```python
from build123d import *

# Parameters (mm, degrees)
EXTRUDE_THIN1_DEPTH = 285.75
FILLET1_R           = 0.889


with BuildPart() as part:
    # Sketch1 → Extrude-Thin1 (new body)
    with BuildSketch(Plane.XY):
        with BuildLine():
            Line((-0.396875, -9.525), (0, -14.2875))
            ThreePointArc((0, -14.2875), (-2.898897336, -13.767099717), (-5.435779046, -12.270886692))
            ThreePointArc((-5.435779046, -12.270886692), (-8.464256404, -10.6095065), (-11.90625, -10.31875))
            Line((-11.90625, -10.31875), (-11.90625, -8.73125))
            Line((-11.90625, -8.73125), (-14.2875, -8.73125))
            Line((-14.2875, -8.73125), (-14.2875, -4.7625))
            Line((-14.2875, -4.7625), (-1.285875, -5.55625))
            Line((-1.285875, -5.55625), (-1.285875, 5.55625))
            Line((-1.285875, 5.55625), (-14.2875, 4.7625))
            Line((-14.2875, 4.7625), (-14.2875, 8.73125))
            Line((-14.2875, 8.73125), (-11.90625, 8.73125))
            Line((-11.90625, 8.73125), (-11.90625, 10.31875))
            ThreePointArc((-11.90625, 10.31875), (-8.464256404, 10.6095065), (-5.435779046, 12.270886692))
            ThreePointArc((-5.435779046, 12.270886692), (-2.898897336, 13.767099717), (0, 14.2875))
            Line((0, 14.2875), (-0.396875, 9.525))
            Line((-0.396875, 9.525), (-1.282804179, 9.598827432))
            Line((-1.282804179, 9.598827432), (-0.971469005, 13.334849518))
            ThreePointArc((-0.971469005, 13.334849518), (-3.040522473, 12.749361604), (-4.855962615, 11.596992112))
            ThreePointArc((-4.855962615, 11.596992112), (-7.731844672, 9.916114382), (-11.01725, 9.366424127))
            Line((-11.01725, 9.366424127), (-11.01725, 7.84225))
            Line((-11.01725, 7.84225), (-13.3985, 7.84225))
            Line((-13.3985, 7.84225), (-13.3985, 5.707428664))
            Line((-13.3985, 5.707428664), (-0.396875, 6.501178664))
            Line((-0.396875, 6.501178664), (-0.396875, -6.501178664))
            Line((-0.396875, -6.501178664), (-13.3985, -5.707428664))
            Line((-13.3985, -5.707428664), (-13.3985, -7.84225))
            Line((-13.3985, -7.84225), (-11.01725, -7.84225))
            Line((-11.01725, -7.84225), (-11.01725, -9.366424127))
            ThreePointArc((-11.01725, -9.366424127), (-7.731844672, -9.916114382), (-4.855962615, -11.596992112))
            ThreePointArc((-4.855962615, -11.596992112), (-3.040522473, -12.749361604), (-0.971469005, -13.334849518))
            Line((-0.971469005, -13.334849518), (-1.282804179, -9.598827432))
            Line((-1.282804179, -9.598827432), (-0.396875, -9.525))
        make_face()
    extrude(amount=-EXTRUDE_THIN1_DEPTH)

    # Fillet1
    fillet1_edges = [part.edges().sort_by_distance(p)[0] for p in [
        (-11.90625, -10.31875, -142.875),
        (-14.2875, -8.73125, -142.875),
        (-14.2875, -4.7625, -142.875),
        (-14.2875, 4.7625, -142.875),
        (-14.2875, 8.73125, -142.875),
        (-11.90625, 10.31875, -142.875),
        (-11.01725, 7.84225, -142.875),
        (-0.396875, 6.501178664, -142.875),
        (-0.396875, -6.501178664, -142.875),
        (-11.01725, -7.84225, -142.875),
    ]]
    fillet(fillet1_edges, radius=FILLET1_R)


solid = part.part
```
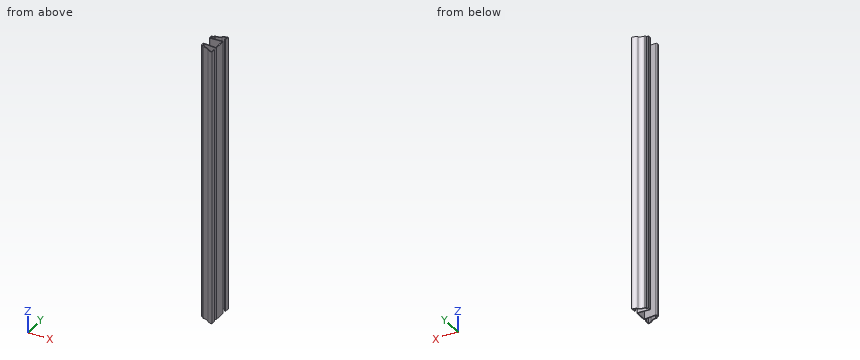
The listing builds one solid part. Answer for the finished solid, in the listing's coordinates (mm). Coordinates: 2 decimals unless noted, no trailing zeros. Order: outer loops, then holes, each group sorted by start corner. A loop starts at its lowest first (then second) coordinate and runs counter-clockwise, first axis right, second up. Notation, with made-up numbers: M -39.5,-35.5 L -26.5,-35.5 A14 ccw -26.5,-13.5 Z; hole C -32,-27.5 d2. An arc over 180 degrees is marked long. Answer as a JSON object with one key per item and string values. Group by question number.
1. Straight lines are drawn through the part: line 1 (Y direction, x = -3, z = -49.5); line 2 (Y direction, x = -2.25, z = -127.5); line 3 (X direction, y = 9, z = -29.5). For each, find the intervals that lie inside material, in ascending order.
2. Flat-ended cylindrical pins translate along their axes: P1, Ø8, axis at y = 3, z = -56.5, coming from the +X side; P2, Ø1.1, axis at y = 6.5, z = -122, coming from the +X side; P3, Ø1.2, axis at x = -13, z = -93, coming from the +Y side. Find the tip coordinate at first contact, or state that the pin passes through.
3. Section B-B on y = -0.5 is taken. Write down the section's boundary in (x, z).
4. Section A-A on x = -8.5 is taken. Write down the section's boundary in (y, z).
Values follow:
{
 "1": {"line 1": "-13.73 to -12.77, -6.34 to -5.45, 5.45 to 6.34, 12.77 to 13.73", "line 2": "-13.98 to -13.05, -6.39 to -5.5, 5.5 to 6.39, 13.05 to 13.98", "line 3": "-11.91 to -11.02"},
 "2": {"P1": "x = -0.4", "P2": "x = -0.49", "P3": "y = 8.73"},
 "3": {"outline": "M -1.29,-285.75 L -0.4,-285.75 L -0.4,0 L -1.29,0 Z"},
 "4": {"outline": "M -10.6,-285.75 L -9.68,-285.75 L -9.68,0 L -10.6,0 Z; M -6.01,-285.75 L -5.12,-285.75 L -5.12,0 L -6.01,0 Z; M 5.12,-285.75 L 6.01,-285.75 L 6.01,0 L 5.12,0 Z; M 9.68,-285.75 L 10.6,-285.75 L 10.6,0 L 9.68,0 Z"}
}
